```python
from build123d import *

# Parameters (mm, degrees)
SKETCH1_W          = 3.5
SKETCH1_H          = 5
CUT_EXTRUDE1_DEPTH = 2
SKETCH3_5_R        = 17
CUT_EXTRUDE2_DEPTH = 1


with BuildPart() as part:
    # Sketch1 → Revolve1 (revolve)
    with BuildSketch(Plane(origin=(0, 0, 0), x_dir=(0, 0, -1), z_dir=(1, 0, 0)), mode=Mode.PRIVATE) as revolve1_sk:
        Polygon((-60, 18), (-60, 7), (-58, 7), (-58, 17), (-31, 17), (-31, 18), (-34.5, 18), align=None)
        with Locations((-32.75, 20.5)):
            Rectangle(SKETCH1_W, SKETCH1_H)
        with Locations((-29.25, 20.5)):
            Rectangle(SKETCH1_W, SKETCH1_H)
        Polygon((-31, 18), (-31, 17), (-2, 17), (-2, 13), (0, 13), (0, 18), (-27.5, 18), align=None)
    revolve(revolve1_sk.sketch.rotate(Axis((0, 0, 1072.381477522), (0, 0, -1)), 90), axis=Axis((0, 0, 1072.381477522), (0, 0, -1)))

    # Sketch3 → Cut-Extrude1 (cut, symmetric)
    with BuildSketch(Plane.XY.offset(31)):
        with BuildLine():
            ThreePointArc((-6.498382723, 17.854159795), (0, -19), (6.498382723, 17.854159795))
            Line((6.498382723, 17.854159795), (7.524443153, 20.673237657))
            ThreePointArc((7.524443153, 20.673237657), (0, 22), (-7.524443153, 20.673237657))
            Line((-7.524443153, 20.673237657), (-6.498382723, 17.854159795))
        make_face()
        with BuildLine():
            add(Edge.make_bspline(
                [(-1, 19.972475891), (-1.837517439, 19.972475891), (-3.400702548, 17.606617047), (-4.505243001, 16.51810785)],
                knots=[0, 0, 0, 0, 1, 1, 1, 1], degree=3))
            Line((-1, 19.972475891), (1, 19.972475891))
            add(Edge.make_bspline(
                [(1, 19.972475891), (1.837517439, 19.972475891), (3.400702548, 17.606617047), (4.505243001, 16.51810785)],
                knots=[0, 0, 0, 0, 1, 1, 1, 1], degree=3))
            Line((4.505243001, 16.51810785), (4.683957663, 16.341987046))
            ThreePointArc((4.683957663, 16.341987046), (13.576215973, 10.231635249), (17, 0))
            ThreePointArc((17, 0), (-10.231635249, -13.576215973), (-4.683957663, 16.341987046))
            Line((-4.683957663, 16.341987046), (-4.505243001, 16.51810785))
        make_face(mode=Mode.SUBTRACT)
    extrude(amount=CUT_EXTRUDE1_DEPTH, both=True, mode=Mode.SUBTRACT)

    # Sketch3_5 → Cut-Extrude2 (cut, symmetric)
    with BuildSketch(Plane.XY.offset(31)):
        Circle(SKETCH3_5_R)
        with BuildLine():
            Line((1, 19.972475891), (-1, 19.972475891))
            add(Edge.make_bspline(
                [(-1, 19.972475891), (-1.837517439, 19.972475891), (-3.400702548, 17.606617047), (-4.505243001, 16.51810785)],
                knots=[0, 0, 0, 0, 1, 1, 1, 1], degree=3))
            Line((-4.505243001, 16.51810785), (-4.683957663, 16.341987046))
            ThreePointArc((-4.683957663, 16.341987046), (0, 17), (4.683957663, 16.341987046))
            Line((4.683957663, 16.341987046), (4.505243001, 16.51810785))
            add(Edge.make_bspline(
                [(1, 19.972475891), (1.837517439, 19.972475891), (3.400702548, 17.606617047), (4.505243001, 16.51810785)],
                knots=[0, 0, 0, 0, 1, 1, 1, 1], degree=3))
        make_face()
        with BuildLine():
            Line((7.524443153, 20.673237657), (6.498382723, 17.854159795))
            ThreePointArc((6.498382723, 17.854159795), (0, -19), (-6.498382723, 17.854159795))
            Line((-6.498382723, 17.854159795), (-7.524443153, 20.673237657))
            ThreePointArc((-7.524443153, 20.673237657), (-12.6186816, -18.021344974), (22, 0))
            ThreePointArc((22, 0), (18.021344974, 12.6186816), (7.524443153, 20.673237657))
        make_face()
    extrude(amount=CUT_EXTRUDE2_DEPTH, both=True, mode=Mode.SUBTRACT)


solid = part.part
```
Read the model definition and answer for the solid it produces. Units are mm, in the model's axes. A direction names the side the tool comes from. Coordinates: 2 decimals unless noted, no trailing zeros. Write each loop counter-clockwise with the first axis right and the second up, starting at its lowest first coordinate (ties: lowest second). Pieces come first, ordered by that corner, then holes. Notation, with made-up numbers: (68.25, -2.5) -> (120.25, -2.5) arc R31 cw to (120.25, 31.5) -> close; hole circle Ø9 at (23, 71). An arc over 180 degrees is marked (long way). Write item = value, one per line.
(1) Straight lines are drawn through the part: L1, parallel to Z at x = 19.5, y = 4; L2, parallel to Z at x = -2, y = -15.5; L3, parallel to Y at x = -0.5, z = 28. For each, find the intervals that lie inside material, in ascending order. Write a range as from..to.
From the geometry:
L1 = 27.5..30, 32..34.5
L2 = 0..2, 58..60
L3 = -22.99..-16.99, 16.99..22.99
(2) Section B-B on z = 41 is taken. Write down the section's boundary in (x, y).
From the geometry:
outline = circle Ø36 at (0, 0); hole circle Ø34 at (0, 0)
(3) Given pin 1 Ø6 at (x, z) = (0, 25) entering from -Y; pin 2 Ø3 at (x, z) = (-1, 39) entering from -Y; pin 3 Ø0.8 at (x, z) = (0.5, 29.5) entering from +Y, each flat-ended and moving along its own axis, determine where each tip first touches the part or whether it passes through.
From the geometry:
pin_1 = -23
pin_2 = -18
pin_3 = 23
(4) Section A-A on x = -20 is taken. Write down the section's boundary in (y, z), plus the area to 3 significant figures.
From the geometry:
outline = (-11.36, 27.5) -> (11.36, 27.5) -> (11.36, 34.5) -> (-11.36, 34.5) -> close; hole (-9.17, 30) -> (9.17, 30) -> (9.17, 32) -> (-9.17, 32) -> close
area = 122 mm2
(5) Which of the six approach directions +Z, -Z, +X, -X, +Y, -Y give full straight-line access (tool end or side, diameter ignored) to faces 1 (the face through (3.23, 6.21, 58.99)), 2 (the face through (15.704, 6.511, 44.818)), 3 (the face through (14, 12, 34.5)), 4 (the face through (14, 12, 27.5))?
From the geometry:
face_1 = +Z, -Z
face_2 = none
face_3 = +Z
face_4 = -Z
(6) For a pull along X with two mould halves and no side action, classify faces 5 (the face through (0, 8, 60)), 6 (the face through (-0.743, -18.985, 32.507)), 7 (the face through (-9, 15, 33)), 8 (the face through (-2.994, -22.804, 31.049)) as +X half, -X half, draft (parallel to the pull), parting line (faces both ways), or undercut.
From the geometry:
face_5 = draft
face_6 = undercut
face_7 = undercut
face_8 = parting line
